Can you work these out from the drawing? Everything is in mm from the part's minimum corner. A direction names the side the tool comes from. Round coordinates to 2 decimals unless told otherwise and drop trailing zeros. Write each loop counter-clockwise with the first axis right and the second up, starting at its lowest first coordinate (ties: lowest second). Pieces come first, ordered by that corner, then holes.
Q1. For the marked faces 4 and 5, which set-ups out of +Z, -Z, +X, -X, +Y, -Y let a thin tool reach every point of the face, with its end or its side?
Q2. If we section it at D-D (x = 23): Please give me the cut outline in (y, z), plus the area to 3 significant figures.
Q3. If we section it at B-B (y = 11): Please give me the cut outline in (x, z).
Q4. I'm going to push flat-ended pins straight in: pin 1 Ø6 at (y, z) = (54.5, 60) entering from +X (1 decimal); pin 2 Ø4 at (y, z) = (69.5, 33) entering from +X; pin 3 Ø7.5 at (x, y) = (56.5, 40.6) entering from -Z; pin 4 Ø12 at (y, z) = (63, 48) entering from +X. Where does each tip first touch, or does it pass through?
Q5. If we section it at C-C (z = 20): Please give me the cut outline in (x, y), plus the area to 3 significant figures.
Q6. Please list where these lines run through material, in increasing order: line 1 along Z through (x, y) = (36.5, 6.5); line 2 along X through (y, z) = (40.6, 89); line 3 along Y through (x, z) = (15, 57.5).
Q7. We'd pull the mould along Z, two halves only. Please class the marked faces 1, 2 and 3: +Z half, -Z half, draft (parallel to the pull), parting line (faces both ways), or undercut.
Q8. If we section it at A-A (x = 56.5): Please give me the cut outline in (y, z), plus the area to 3 significant figures.
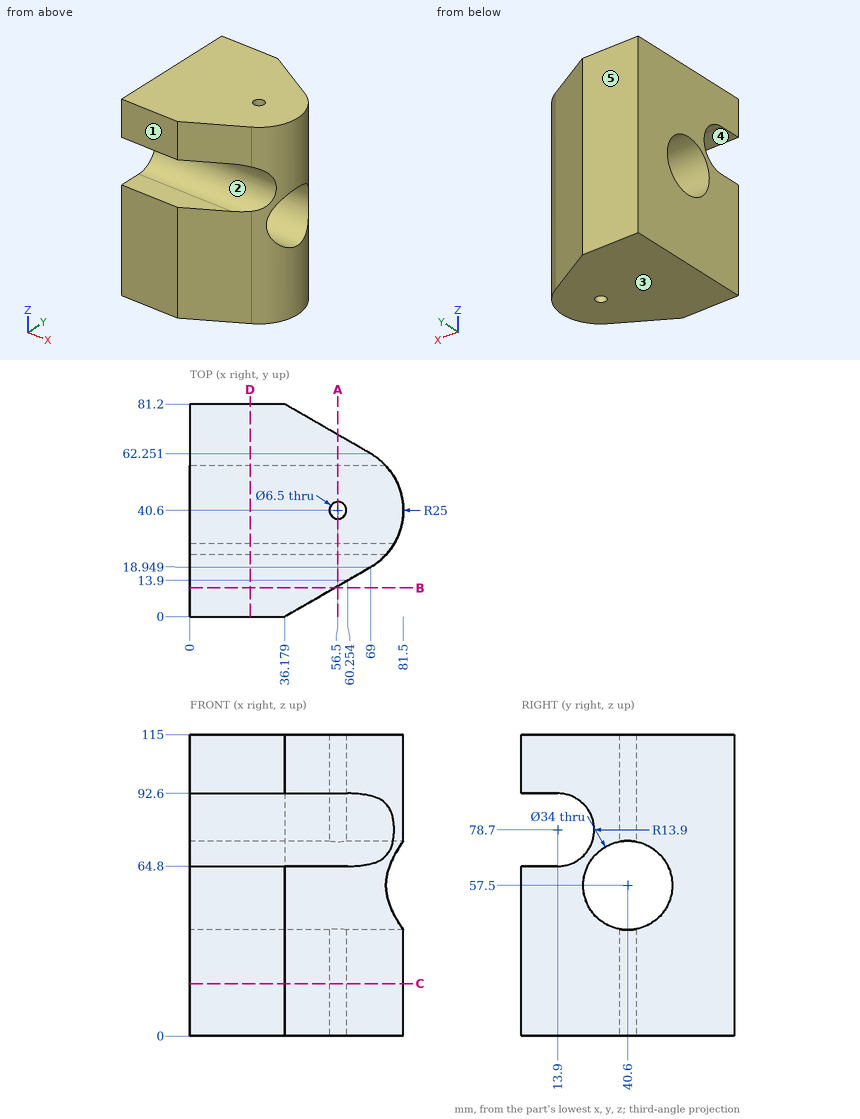
A:
1. face 4: +X, -X, -Y
1. face 5: +Z, -Z, +X, -X, +Y
2. outline: (0, 0) - (81.2, 0) - (81.2, 115) - (0, 115) - (0, 92.6) - (13.9, 92.6) arc R13.9 cw to (13.9, 64.8) - (0, 64.8) - close; hole circle Ø34 at (40.6, 57.5)
2. area: 7,740 mm2
3. outline: (0, 0) - (55.23, 0) - (55.23, 64.8) - (0, 64.8) - close; (0, 92.6) - (55.23, 92.6) - (55.23, 115) - (0, 115) - close
4. pin 1: stops at x = 75.2
4. pin 2: stops at x = 59.91
4. pin 3: stops at z = 0
4. pin 4: stops at x = 75.37
5. outline: (0, 0) - (36.18, 0) - (69, 18.95) arc R25 ccw to (69, 62.25) - (36.18, 81.2) - (0, 81.2) - close; hole circle Ø6.5 at (56.5, 40.6)
5. area: 5,330 mm2
6. line 1: z = 0 to 64.8, 92.6 to 115
6. line 2: x = 0 to 53.25, 59.75 to 81.5
6. line 3: y = 0 to 23.6, 57.6 to 81.2
7. face 1: draft
7. face 2: undercut
7. face 3: -Z half
8. outline: (11.73, 0) - (37.35, 0) - (37.35, 40.81) arc R17 cw to (37.35, 74.19) - (37.35, 115) - (11.73, 115) - (11.73, 92.6) - (13.9, 92.6) arc R13.9 cw to (13.9, 64.8) - (11.73, 64.8) - close; (43.85, 0) - (69.47, 0) - (69.47, 115) - (43.85, 115) - (43.85, 74.19) arc R17 cw to (43.85, 40.81) - close
8. area: 4,840 mm2
